For this review, take the finished solid that the model builds, in its own axes (mm). Coordinates: 2 decimals unless noted, no trailing zeros. Loops run counter-clockwise (first coordinate to the right, second up) from the corner with the lowest first, then second, coordinate; pieces in that order, holes last.
1. Clearance check with flat-ended pins moving along their axes: P1, Ø8, axis at y = 3.5, z = -33.5, coming from the +X side; P2, Ø3, axis at x = 110.5, y = 11.5, coming from the +Z side; P3, Ø14, axis at x = 152, z = 3.5, coming from the +Y side; P4, Ø4, axis at x = -1.5, z = 146.5, coming from the +Y side. State where each tip first meets the part, or that it passes through.
2. Take a section at C-C, the plane z = -73. State the section outline as (x, y) points, then the cut area to 3 significant figures.
3. Take a section at B-B, the plane x = 77.5. State the section outline as (y, z) points.
4. Take a section at A-A, the plane y = 10.75. State the section outline as (x, z) points.
5. To check wall thickness, follow probe 1 along Z at (x, y) = (-13.5, 13.5); probe 2 along X at (y, z) = (14.75, 2); probe 3 along Z at (x, y) = (126.5, 6). State the ranges of each line that lie inside material, in increasing order.
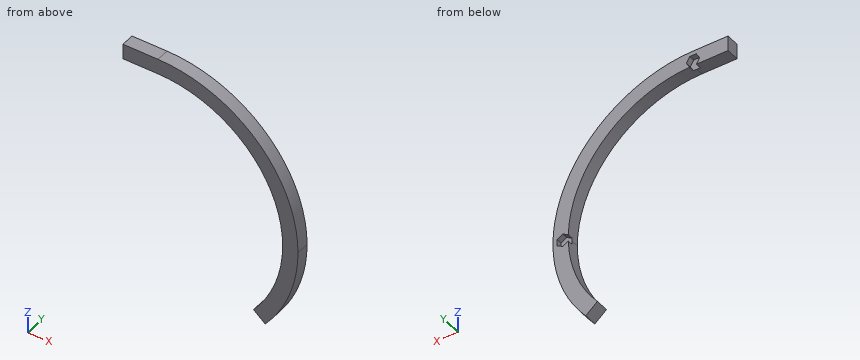
```python
from build123d import *

# Parameters (mm, degrees)
BOSS_EXTRUDE1_DEPTH = 15
SKETCH2_W           = 17.5
SKETCH2_H           = 15
BOSS_EXTRUDE2_DEPTH = 40
CUT_EXTRUDE1_DEPTH  = 6.5


with BuildPart() as part:
    # Sketch1 → Boss-Extrude1 (new body)
    with BuildSketch(Plane(origin=(0, 0, 0), x_dir=(1, 0, 0), z_dir=(0, 1, 0))):
        with BuildLine():
            ThreePointArc((142.5, 0), (100.762716319, -100.762716319), (0, -142.5))
            Line((0, -142.5), (0, -160))
            ThreePointArc((0, -160), (113.13708499, -113.13708499), (160, 0))
            ThreePointArc((160, 0), (150.350819326, 54.723222932), (122.567110899, 102.84601755))
            Line((122.567110899, 102.84601755), (109.161333144, 91.59723438))
            ThreePointArc((109.161333144, 91.59723438), (133.906198462, 48.737870424), (142.5, 0))
        make_face()
    extrude(amount=BOSS_EXTRUDE1_DEPTH)

    # Sketch2 → Boss-Extrude2 (add)
    with BuildSketch(Plane.ZY):
        with Locations((151.25, 7.5)):
            Rectangle(SKETCH2_W, SKETCH2_H)
    extrude(amount=BOSS_EXTRUDE2_DEPTH)

    # Sketch3 → Cut-Extrude1 (cut)
    with BuildSketch(Plane(origin=(0, 15, 0), x_dir=(1, 0, 0), z_dir=(0, 1, 0))):
        Polygon((-3.75277675, -142.2), (-7.505553499, -148.7), (-3.75277675, -155.2), (3.75277675, -155.2), (7.505553499, -148.7), (3.75277675, -142.2), align=None)
        Polygon((142.2, 3.75277675), (142.2, -3.75277675), (148.7, -7.505553499), (155.2, -3.75277675), (155.2, 3.75277675), (148.7, 7.505553499), align=None)
    extrude(amount=-CUT_EXTRUDE1_DEPTH, mode=Mode.SUBTRACT)


solid = part.part
```
Results list:
1. P1: stops at x = 157.26
1. P2: stops at z = 117.13
1. P3: stops at y = 15
1. P4: stops at y = 8.5
2. outline: (122.38, 0) - (142.38, 0) - (142.38, 15) - (122.38, 15) - close
2. area: 300 mm2
3. outline: (0, 119.58) - (15, 119.58) - (15, 139.98) - (0, 139.98) - close
4. outline: (-40, 142.5) - (-3.93, 142.5) - (-7.51, 148.7) - (-3.75, 155.2) - (3.75, 155.2) - (7.51, 148.7) - (3.9, 142.45) arc R142.5 cw to (142.45, 3.9) - (148.7, 7.51) - (155.2, 3.75) - (155.2, -3.75) - (148.7, -7.51) - (142.45, -3.9) arc R142.5 cw to (109.16, -91.6) - (122.57, -102.85) arc R160 ccw to (0, 160) - (-40, 160) - close
5. probe 1: z = 142.5 to 160
5. probe 2: x = 155.2 to 159.99
5. probe 3: z = -97.97 to -65.6, 65.6 to 97.97
